Source: CAD feature listing. Evaluate the final solid. Frame: model axes, mm. A direction names the side the tool comes from. Give positions to 0.01 mm unless a question says otherwise; leave off trailing zeros. Order: outer loops, then holes, each group sorted by start corner. A loop starts at its lowest first (then second) coordinate and runs counter-clockwise, first axis right, second up. Notation, with made-up numbers: M 4,63 L 59,63 A7 cw 59,68 Z; hole C -18,5.25 d7. An arc over 180 degrees is marked long. Use CSV: the item, a comma, the result in double quotes. Start each with the question number.
Item 1: Section query B-B on x = 0. Return loops of the section in (y, z).
Item 2: Ray query, probe 1 along X at (y, z) = (3, 2); probe 2 along X at (y, z) = (15.25, 1); probe 3 along Y at (x, z) = (1.5, -2.25). Return the intervals inside material, ascending. Write a range as from..to.
Item 3: Access query for faces 1 (the face through (0, 15, 2)), 2 (the face through (-1.74, 14.88, 0.99)), 3 (the face through (1.724, 14.878, 1.014)), 4 (the face through (-1.724, 14.878, -1.014)), 5 (the face through (1.74, 14.88, -0.99)). Directions: +Z, -Z, +X, -X, +Y, -Y. A direction counts if a zero-diameter tool reaches every point of the face in a straight line with its end or side. Return the directions, or none.
Item 4: Section query C-C on y = 7. Return loops of the section in (x, z), and give its area (3 significant figures).
Item 5: Section query A-A on y = 15.5. Return loops of the section in (x, z).
Item 6: Pull-direction query (X, two-part tool) for faces 6 (the face through (-1.775, 12.663, -1.043)), 7 (the face through (0, 15, -2)), 8 (the face through (1.775, 12.663, 1.043)); classes: +X half, -X half, draft (parallel to the pull), parting line (faces both ways), or undercut.
Item 7: First-contact query: pin 1 (1.5 mm diameter, centred on x = 0, z = -1.5, fed in from -Y); pin 2 (3 mm diameter, centred on y = 3.5, z = -2, fed in from -X); pin 3 (0.7 mm diameter, centred on x = 0, y = 15.5, fed in from +Z); pin 4 (2.5 mm diameter, centred on x = 0, y = 15.5, fed in from -Z). Flat tips, straight axial feed; report the tip coordinate or a pass-through.
from build123d import *

# Parameters (mm, degrees)
BOSS_EXTRUDE1_DEPTH = 13
BOSS_EXTRUDE2_DEPTH = 4
SKETCH8_R           = 1
CUT_EXTRUDE1_DEPTH  = 4.464101715
CIRPATTERN1_COUNT   = 6


with BuildPart() as part:
    # Sketch2 → Boss-Extrude1 (new body)
    with BuildSketch(Plane(origin=(0, 0, 0), x_dir=(1, 0, 0), z_dir=(0, 1, 0))):
        Polygon((3.464101615, 0), (1.732050808, 3), (-1.732050808, 3), (-3.464101615, 0), (-1.732050808, -3), (1.732050808, -3), align=None)
    extrude(amount=BOSS_EXTRUDE1_DEPTH)

    # Sketch3 → Boss-Extrude2 (add)
    with BuildSketch(Plane(origin=(0, 13, 0), x_dir=(1, 0, 0), z_dir=(0, 1, 0))):
        Polygon((2.309401077, 0), (1.154700538, 2), (-1.154700538, 2), (-2.309401077, 0), (-1.154700538, -2), (1.154700538, -2), align=None)
    extrude(amount=BOSS_EXTRUDE2_DEPTH)

    # Sketch5 → Cut-Revolve2 (revolve, cut)
    with BuildSketch(Plane.XY):
        Polygon((3.464101615, 1), (2.464101615, 0), (3.464101615, 0), align=None)
        Polygon((1.809401077, 17), (2.309401077, 16.5), (2.309401077, 17), align=None)
        with BuildLine():
            Line((2.309401077, 13), (3.464101615, 13))
            Line((3.464101615, 13), (3.464101615, 9.990187462))
            ThreePointArc((3.464101615, 9.990187462), (2.607981818, 11.388145102), (2.309401077, 13))
        make_face()
    revolve(axis=Axis((0, 17, 0), (0, -1, 0)), mode=Mode.SUBTRACT)

    # Sketch8 → Cut-Extrude1 (cut, symmetric)
    with BuildSketch(Plane(origin=(0, 0, 0), x_dir=(0, 0, -1), z_dir=(1, 0, 0))):
        with Locations((3, 13)):
            Circle(SKETCH8_R)
    cut_extrude1 = extrude(amount=CUT_EXTRUDE1_DEPTH, both=True, mode=Mode.SUBTRACT)

    # CirPattern1: Cut-Extrude1 ×6 about axis
    cirpattern1_axis = Axis((0, 17, 0), (0, 1, 0))
    for i in range(1, CIRPATTERN1_COUNT):
        add(cut_extrude1.rotate(cirpattern1_axis, i * 360 / CIRPATTERN1_COUNT), mode=Mode.SUBTRACT)


solid = part.part
Verdict:
1,outline,"M 0,-2.46 L 0.54,-3 L 10.6,-3 A4.5 cw 12.22,-2.38 A1 cw 13,-2 L 16.81,-2 L 17,-1.81 L 17,1.81 L 16.81,2 L 13,2 A1 cw 12.22,2.38 A4.5 cw 10.6,3 L 0.54,3 L 0,2.46 Z"
2,probe 1,"-2.31..2.31"
2,probe 2,"-1.73..1.73"
2,probe 3,"0.24..11.16"
3,face 1,"+Z, +X, -X, +Y"
3,face 2,"+Z, -X, +Y"
3,face 3,"+Z, +X, +Y"
3,face 4,"-Z, -X, +Y"
3,face 5,"-Z, +X, +Y"
4,outline,"M -3.46,0 L -1.73,-3 L 1.73,-3 L 3.46,0 L 1.73,3 L -1.73,3 Z"
4,area,"31.2 mm2"
5,outline,"M -2.31,0 L -1.15,-2 L 1.15,-2 L 2.31,0 L 1.15,2 L -1.15,2 Z"
6,face 6,"-X half"
6,face 7,"draft"
6,face 8,"+X half"
7,pin 1,"y = 0"
7,pin 2,"x = -3.18"
7,pin 3,"z = 2"
7,pin 4,"z = -2"
